from build123d import *

# Parameters (mm, degrees)
SKETCH1_W           = 25
SKETCH1_H           = 25
SKETCH1_R           = 3
BOSS_EXTRUDE1_DEPTH = 200
SKETCH2_R           = 2.5
CUT_EXTRUDE1_DEPTH  = 26


with BuildPart() as part:
    # Sketch1 → Boss-Extrude1 (new body)
    with BuildSketch(Plane(origin=(0, 0, 0), x_dir=(1, 0, 0), z_dir=(0, 1, 0))):
        with Locations((-7.413793103, -2.327586207)):
            Rectangle(SKETCH1_W, SKETCH1_H)
        with Locations((-7.413793103, -2.327586207)):
            Circle(SKETCH1_R, mode=Mode.SUBTRACT)
    extrude(amount=BOSS_EXTRUDE1_DEPTH)

    # Sketch2 → Cut-Extrude1 (cut, through all)
    with BuildSketch(Plane.XY.offset(14.827586207)):
        with Locations((-7.413793103, 190)):
            Circle(SKETCH2_R)
    extrude(amount=-CUT_EXTRUDE1_DEPTH, mode=Mode.SUBTRACT)


solid = part.part
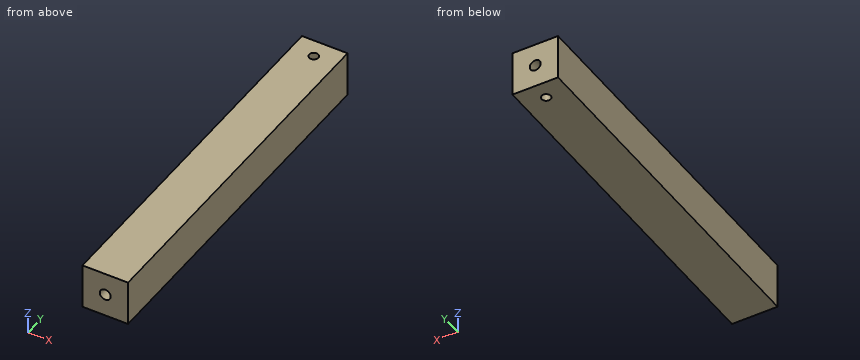
Model file for the job. Use its own axes, mm. Round coordinates to 2 decimals unless told otherwise and drop trailing zeros. Order: outer loops, then holes, each group sorted by start corner. A loop starts at its lowest first (then second) coordinate and runs counter-clockwise, first axis right, second up. Notation, with made-up numbers: M 70.25,81.25 L 116.25,81.25 A7 cw 116.25,92.25 Z; hole C -37.5,36 d1. An arc over 180 degrees is marked long. Write each question's results on one line, items separated by ' | '. Start each with the question number.
(1) Saw through at B-B, the plane y = 25. Give the cut face in (x, z).
(2) Probe probe 1 along X at (y, z) = (190, -2.5); probe 2 along X at (y, z) = (126, 2.25); probe 3 along Y at (x, z) = (-7, -4). List the from-to ranges inside material, lowest first. Write a range as from..to.
(3) Saw through at A-A, the plane y = 190. Give the cut face in (x, z).
Established:
1) outline: M -19.91,-10.17 L 5.09,-10.17 L 5.09,14.83 L -19.91,14.83 Z; hole C -7.41,2.33 d6
2) probe 1: x = -19.91..-9.91, -4.91..5.09 | probe 2: x = -19.91..-10.41, -4.41..5.09 | probe 3: y = 0..187.53, 192.47..200
3) outline: M -19.91,-10.17 L -9.91,-10.17 L -9.91,0.67 A3 cw -9.91,3.99 L -9.91,14.83 L -19.91,14.83 Z; M -4.91,-10.17 L 5.09,-10.17 L 5.09,14.83 L -4.91,14.83 L -4.91,3.99 A3 cw -4.91,0.67 Z
